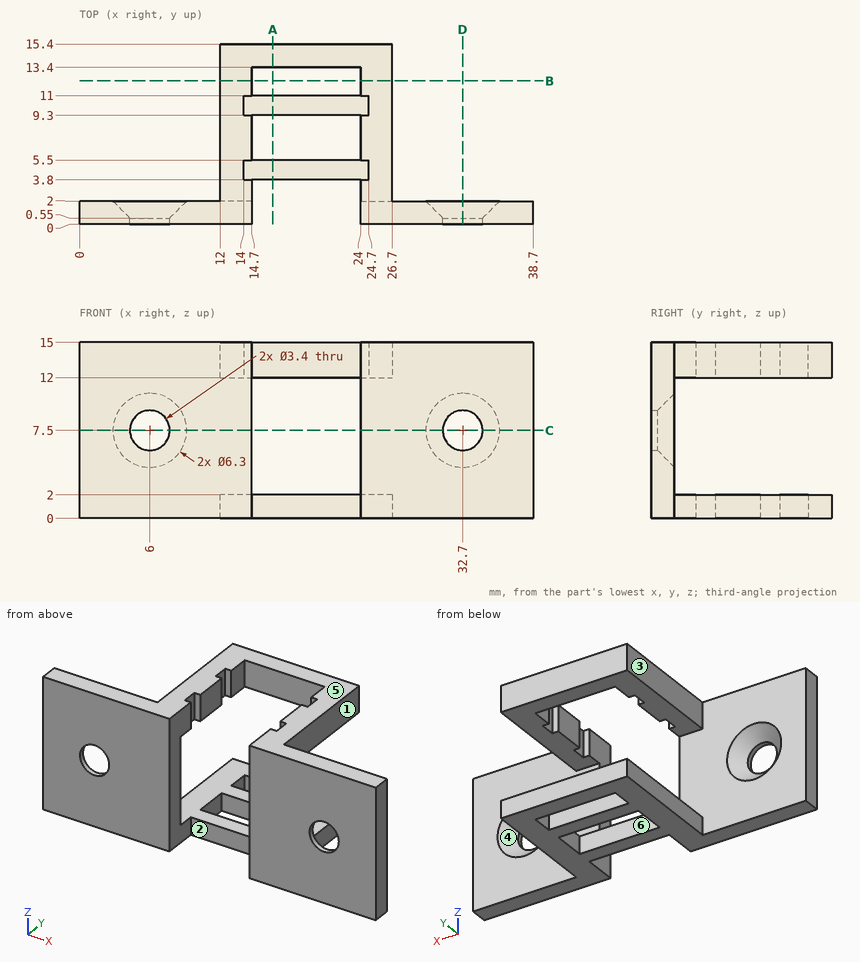
Study the drawing (mm; zero at the part's minimum x, y, z) and answer. A direction names the side the tool comes from. Round coordinates to 2 decimals unless told otherwise and drop trailing zeros. Loops run counter-clockwise (first coordinate to the right, second up) from the corner with the lowest first, then second, coordinate; pieces in that order, holes last.
Q1. For a pull along Z with two mould halves and no side action, classify the marked faces 4, 5 and 6 as released by +Z, released by -Z, zero draft, split by the parting line, or undercut.
Q2. Find the intervals of material crossed by line 1 (Y direction, x = 20.5, z = 1.75); line 2 (X direction, y = 0.3, z = 7.5); line 3 (Z direction, x = 32.7, y = 0.25), in increasing order.
Q3. Section A-A, the plane x = 16.5 is taken. Determine the outline of the cut face in (y, z), then the cut area to 3 significant figures.
Q4. Section D-D, the plane x = 32.7 is taken. Determine the outline of the cut face in (y, z), then the cut area to 3 significant figures.
Q5. Section C-C, the plane z = 7.5 is taken. Determine the outline of the cut face in (x, y), then the cut area to 3 significant figures.
Q6. Section B-B, the plane y = 12.25 is taken. Determine the outline of the cut face in (x, z).
Q7. Given pin 1 Ø4 at (x, y) = (18.5, 9.5) entering from +Z; pin 2 Ø0.5 at (y, z) = (10, 13.5) entering from +X; pin 3 Ø1.5 at (x, z) = (19, 13.5) entering from -Y; pin 4 Ø2 at (y, z) = (11.5, 4.5) entering from -X, each flat-ended and moving along its own axis, determine where each tip first touches the part or whether it passes through.
Q8. Which of the six approach directions +Z, -Z, +X, -X, +Y, -Y give full straight-line access (tool end or side, diameter ignored) to the marked faces 1, 2 and 3?
Completed:
1. face 4: undercut
1. face 5: released by +Z
1. face 6: zero draft
2. line 1: y = 3.8 to 5.5, 9.3 to 11, 13.4 to 15.4
2. line 2: x = 0 to 4.3, 7.7 to 14.7, 24 to 31, 34.4 to 38.7
2. line 3: z = 0 to 5.8, 9.2 to 15
3. outline: (3.8, 0) - (5.5, 0) - (5.5, 2) - (3.8, 2) - close; (9.3, 0) - (11, 0) - (11, 2) - (9.3, 2) - close; (13.4, 0) - (15.4, 0) - (15.4, 2) - (13.4, 2) - close; (13.4, 12) - (15.4, 12) - (15.4, 15) - (13.4, 15) - close
3. area: 16.8 mm2
4. outline: (0, 0) - (2, 0) - (2, 4.35) - (0.55, 5.8) - (0, 5.8) - close; (0, 9.2) - (0.55, 9.2) - (2, 10.65) - (2, 15) - (0, 15) - close
4. area: 21.1 mm2
5. outline: (0, 0) - (4.3, 0) - (4.3, 0.55) - (2.85, 2) - (0, 2) - close; (7.7, 0) - (14.7, 0) - (14.7, 2) - (9.15, 2) - (7.7, 0.55) - close; (24, 0) - (31, 0) - (31, 0.55) - (29.55, 2) - (24, 2) - close; (34.4, 0) - (38.7, 0) - (38.7, 2) - (35.85, 2) - (34.4, 0.55) - close
5. area: 41.0 mm2
6. outline: (12, 0) - (14.7, 0) - (14.7, 2) - (12, 2) - close; (12, 12) - (14.7, 12) - (14.7, 15) - (12, 15) - close; (24, 0) - (26.7, 0) - (26.7, 2) - (24, 2) - close; (24, 12) - (26.7, 12) - (26.7, 15) - (24, 15) - close
7. pin 1: stops at z = 2
7. pin 2: stops at x = 26.7
7. pin 3: stops at y = 13.4
7. pin 4: passes through
8. face 1: +Z, -Z, +X, +Y
8. face 2: +Z, -Z, -Y
8. face 3: +Z, -Z, -X, +Y
